from build123d import *

# Parameters (mm, degrees)
SKETCH1_W           = 70
SKETCH1_H           = 47
BOSS_EXTRUDE1_DEPTH = 10
SKETCH2_R           = 11.5
CUT_EXTRUDE1_DEPTH  = 10
SKETCH3_R           = 1.5
CUT_EXTRUDE2_DEPTH  = 10
SKETCH4_R           = 4.05
CUT_EXTRUDE3_DEPTH  = 10
SKETCH6_R           = 2
CUT_EXTRUDE5_DEPTH  = 10
SKETCH7_R           = 3.5
CUT_EXTRUDE6_DEPTH  = 7
CHAMFER1_SIZE       = 10


with BuildPart() as part:
    # Sketch1 → Boss-Extrude1 (new body)
    with BuildSketch(Plane.XY):
        Rectangle(SKETCH1_W, SKETCH1_H)
    extrude(amount=BOSS_EXTRUDE1_DEPTH)

    # Sketch2 → Cut-Extrude1 (cut)
    with BuildSketch(Plane.XY.offset(10)):
        Circle(SKETCH2_R)
    extrude(amount=-CUT_EXTRUDE1_DEPTH, mode=Mode.SUBTRACT)

    # Sketch3 → Cut-Extrude2 (cut)
    with BuildSketch(Plane.XY.offset(10)):
        with Locations((-15.5, 15.5)):
            Circle(SKETCH3_R)
        with Locations((15.5, 15.5)):
            Circle(SKETCH3_R)
        with Locations((15.5, -15.5)):
            Circle(SKETCH3_R)
        with Locations((-15.5, -15.5)):
            Circle(SKETCH3_R)
    extrude(amount=-CUT_EXTRUDE2_DEPTH, mode=Mode.SUBTRACT)

    # Sketch4 → Cut-Extrude3 (cut)
    with BuildSketch(Plane.XY.offset(10)):
        with Locations((-22, 10.5)):
            Circle(SKETCH4_R)
        with Locations((22, 10.5)):
            Circle(SKETCH4_R)
    extrude(amount=-CUT_EXTRUDE3_DEPTH, mode=Mode.SUBTRACT)

    # Sketch6 → Cut-Extrude5 (cut)
    with BuildSketch(Plane.XY.offset(10)):
        with Locations((-27.5, -18.5)):
            Circle(SKETCH6_R)
        with Locations((27.5, -18.5)):
            Circle(SKETCH6_R)
    extrude(amount=-CUT_EXTRUDE5_DEPTH, mode=Mode.SUBTRACT)

    # Sketch7 → Cut-Extrude6 (cut)
    with BuildSketch(Plane.XY.offset(10)):
        with Locations((-15.5, -15.5)):
            Circle(SKETCH7_R)
        with Locations((-15.5, 15.5)):
            Circle(SKETCH7_R)
        with Locations((15.5, 15.5)):
            Circle(SKETCH7_R)
        with Locations((15.5, -15.5)):
            Circle(SKETCH7_R)
    extrude(amount=-CUT_EXTRUDE6_DEPTH, mode=Mode.SUBTRACT)

    # Chamfer1
    chamfer1_edges = [part.edges().sort_by_distance(p)[0] for p in [
        (-35, 23.5, 5),
        (35, 23.5, 5),
    ]]
    chamfer(chamfer1_edges, length=CHAMFER1_SIZE)


solid = part.part
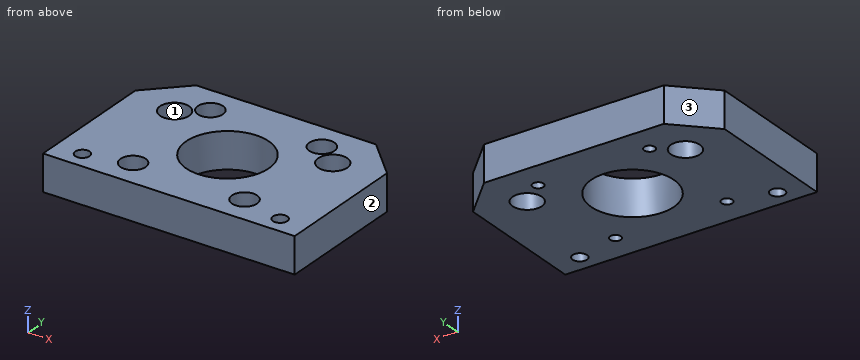
Could you check a few things on this model? Use its own coordinates, in mm. Face numbers are marked on the shaded views. Give positions to 0.01 mm unless a question says otherwise; leave off trailing zeros. Order: outer loops, then holes, each group sorted by start corner. A loop starts at its lowest first (then second) coordinate and runs counter-clockwise, first axis right, second up.
1. Suppose I cut it at C-C (z = 5). State how many separate pieces and enclosed holes the cut face has, plus the area to 3 significant figures.
Answers below:
separate pieces: 1
enclosed holes: 9
area: 2,490 mm2
2. For pin 1 (3.5 mm diameter, centred on x = 17, y = 16, fed in from +Z); pin 2 (5 mm diameter, centred on x = -22, y = 10.5, fed in from -Z), each with a flat end and sliding along its axis, tell me the tip position at first contact or that it passes through.
Answers below:
pin 1: stops at z = 3
pin 2: passes through
3. Suppose I cut it at B-B (x = 27.5). Write out the boundary of the cut face in (y, z), plus the area to 3 significant figures.
Answers below:
outline: (-23.5, 0) - (-20.5, 0) - (-20.5, 10) - (-23.5, 10) - close; (-16.5, 0) - (21, 0) - (21, 10) - (-16.5, 10) - close
area: 405 mm2
4. I need wall thicknesses on L1, parallel to Y at x = 15.5, z = 0.7; L2, parallel to X at y = -0.5, z = 2.5; L3, parallel to Y at x = 0, z = 3.5. Which ranges of each line are inside material? Lowest first, please.
Answers below:
L1: y = -23.5 to -17, -14 to 14, 17 to 23.5
L2: x = -35 to -11.49, 11.49 to 35
L3: y = -23.5 to -11.5, 11.5 to 23.5
5. Suppose I cut it at A-A (y = -15.5). Write out the boundary of the cut face in (x, z), plus the area to 3 significant figures.
Answers below:
outline: (-35, 0) - (-17, 0) - (-17, 3) - (-19, 3) - (-19, 10) - (-35, 10) - close; (-14, 0) - (14, 0) - (14, 3) - (12, 3) - (12, 10) - (-12, 10) - (-12, 3) - (-14, 3) - close; (17, 0) - (35, 0) - (35, 10) - (19, 10) - (19, 3) - (17, 3) - close
area: 584 mm2
6. Suppose I cut it at D-D (y = -9.5). Write out the boundary of the cut face in (x, z), plus the area to 3 significant figures.
Answers below:
outline: (-35, 0) - (-6.48, 0) - (-6.48, 10) - (-35, 10) - close; (6.48, 0) - (35, 0) - (35, 10) - (6.48, 10) - close
area: 570 mm2
7. Thinking about a two-plate mould opening in Y: for the marked faces 1, 2 and 3, which applies, +Y half, -Y half, draft (parallel to the pull), parting line (faces both ways), or undercut?
Answers below:
face 1: undercut
face 2: draft
face 3: +Y half
